from build123d import *

# Parameters (mm, degrees)
SKETCH1_W           = 50
SKETCH1_H           = 49.309999932
BOSS_EXTRUDE1_DEPTH = 22.098
SKETCH3_R           = 2.667
BOSS_EXTRUDE2_DEPTH = 14.098
SKETCH11_R          = 1.5875
CUT_EXTRUDE7_DEPTH  = 33.02
BOSS_EXTRUDE4_DEPTH = 2.54
SKETCH16_R          = 1.5875
CUT_EXTRUDE11_DEPTH = 2.54
BOSS_EXTRUDE5_DEPTH = 7
SKETCH21_R          = 3
CUT_EXTRUDE14_DEPTH = 7
BOSS_EXTRUDE6_DEPTH = 5


with BuildPart() as part:
    # Sketch1 → Boss-Extrude1 (new body)
    with BuildSketch(Plane.XY):
        with Locations((0, 0.745000034)):
            Rectangle(SKETCH1_W, SKETCH1_H)
        Polygon((12.5, 47.050635095), (-12.5, 47.050635095), (-25, 25.4), (25, 25.4), align=None)
    extrude(amount=BOSS_EXTRUDE1_DEPTH)

    # Sketch3 → Boss-Extrude2 (add)
    with BuildSketch(Plane(origin=(0, 0, 0), x_dir=(-1, 0, 0), z_dir=(0, 0, -1))):
        with BuildLine():
            ThreePointArc((-26.155685571, 27.78125), (-33.743775214, 30.924339642), (-30.600685571, 23.33625))
            Line((-30.600685571, 23.33625), (-25, 23.33625))
            Line((-25, 23.33625), (-25, 25.4))
            Line((-25, 25.4), (-23.625184671, 27.78125))
            Line((-23.625184671, 27.78125), (-26.155685571, 27.78125))
        make_face()
        with Locations((-30.600685571, 27.78125)):
            Circle(SKETCH3_R, mode=Mode.SUBTRACT)
    extrude(amount=-BOSS_EXTRUDE2_DEPTH)

    # Sketch11 → Cut-Extrude7 (cut)
    with BuildSketch(Plane.XY.offset(22.098)):
        with BuildLine():
            Line((-17.892329478, 22.025071278), (-19.92, 22.179409051))
            Line((-19.92, 22.179409051), (-19.92, -11.209999932))
            Line((-19.92, -11.209999932), (-18.65, -11.209999932))
            ThreePointArc((-18.65, -11.209999932), (-14.159871939, -13.069871871), (-12.3, -17.559999932))
            Line((-12.3, -17.559999932), (-12.3, -18.829999932))
            Line((-12.3, -18.829999932), (12.3, -18.829999932))
            Line((12.3, -18.829999932), (12.3, -17.559999932))
            ThreePointArc((12.3, -17.559999932), (14.159871939, -13.069871871), (18.65, -11.209999932))
            Line((18.65, -11.209999932), (19.92, -11.209999932))
            Line((19.92, -11.209999932), (19.92, 24.038818102))
            Line((19.92, 24.038818102), (18.060590949, 27.259409051))
            Line((18.060590949, 27.259409051), (9.567060633, 41.970635095))
            Line((9.567060633, 41.970635095), (-9.567060633, 41.970635095))
            Line((-9.567060633, 41.970635095), (-18.024928281, 27.321178603))
            ThreePointArc((-18.024928281, 27.321178603), (-12.880508254, 24.800266004), (-17.892329478, 22.025071278))
        make_face()
        with Locations((-16.11, 24.719409119)):
            Circle(SKETCH11_R)
        with Locations((16.11, -15.02)):
            Circle(SKETCH11_R)
        with Locations((-16.11, -15.019999932)):
            Circle(SKETCH11_R)
    extrude(amount=-CUT_EXTRUDE7_DEPTH, mode=Mode.SUBTRACT)

    # Sketch12 → Boss-Extrude4 (add)
    with BuildSketch(Plane(origin=(0, 0, 0), x_dir=(-1, 0, 0), z_dir=(0, 0, -1))):
        Polygon((-25, -23.909999932), (25, -23.909999932), (25, 25.4), (12.5, 47.050635095), (-12.5, 47.050635095), (-25, 25.4), align=None)
    extrude(amount=-BOSS_EXTRUDE4_DEPTH)

    # Sketch16 → Cut-Extrude11 (cut)
    with BuildSketch(Plane.XY.offset(2.54)):
        with Locations((-10.16, 6.35)):
            Circle(SKETCH16_R)
        with Locations((-10.16, -6.35)):
            Circle(SKETCH16_R)
        with Locations((10.16, 6.35)):
            Circle(SKETCH16_R)
        with Locations((10.16, -6.35)):
            Circle(SKETCH16_R)
    extrude(amount=-CUT_EXTRUDE11_DEPTH, mode=Mode.SUBTRACT)

    # Sketch20 → Boss-Extrude5 (add)
    with BuildSketch(Plane.XY.offset(2.54)):
        Polygon((-9.198279291, 25.191225954), (-6.198279291, 25.191225954), (-6.198279291, 26.191225954), (-8.198279291, 26.191225954), (-8.198279291, 27.391225954), (-6.198279291, 27.391225954), (-6.198279291, 28.391225954), (-9.198279291, 28.391225954), align=None)
        Polygon((8.198279291, 26.191225954), (8.198279291, 27.391225954), (6.198279291, 27.391225954), (6.198279291, 28.391225954), (9.198279291, 28.391225954), (9.198279291, 25.191225954), (6.198279291, 25.191225954), (6.198279291, 26.191225954), align=None)
    extrude(amount=BOSS_EXTRUDE5_DEPTH)

    # Sketch21 → Cut-Extrude14 (cut)
    with BuildSketch(Plane.XY.offset(2.54)):
        with Locations((0.698279291, 30.391225954)):
            Circle(SKETCH21_R)
    extrude(amount=-CUT_EXTRUDE14_DEPTH, mode=Mode.SUBTRACT)

    # Sketch22 → Boss-Extrude6 (add)
    with BuildSketch(Plane.XY.offset(2.54)):
        Polygon((4, 1.5), (-4, 1.5), (-4, 0.5), (-3, 0.5), (3, 0.5), (4, 0.5), align=None)
        Polygon((3, -0.5), (-3, -0.5), (-4, -0.5), (-4, -1.5), (4, -1.5), (4, -0.5), align=None)
    extrude(amount=BOSS_EXTRUDE6_DEPTH)


solid = part.part
Here's how the part is built. I have some questions about the finished solid (model axes, mm). A direction names the side the tool comes from. Round coordinates to 2 decimals unless told otherwise and drop trailing zeros. Order: outer loops, then holes, each group sorted by start corner. A loop starts at its lowest first (then second) coordinate and runs counter-clockwise, first axis right, second up. Notation, with made-up numbers: (-17.5, -4.75) -> (0.5, -4.75) arc R27 ccw to (0.5, 31.25) -> close; hole circle Ø3 at (60.25, 1.25). An arc over 180 degrees is marked (long way). Return JSON: item names as keys, results as strings.
Q1. If we section it at B-B on z = 1.75: Give the number of separate pieces and of enclosed holes in the cut face, plus the area to 3 significant figures.
Filled sheet:
{"separate pieces": "1", "enclosed holes": "6", "area": "3,270 mm^2"}
Q2. If we mould it in two halves opening along Y, with no side actions, what happens to faces 3 (the cylindrical face through (-12.884, 24.899, 12.456)), 4 (the flat face through (0, 47.051, 11))? For each: released by +Y, released by -Y, zero draft, split by the parting line, or undercut.
Filled sheet:
{"face 3": "undercut", "face 4": "released by +Y"}
Q3. If we section it at C-C on y = 10.5: List the corners of the cut face in (x, z) for me, plus the area to 3 significant figures.
Filled sheet:
{"outline": "(-25, 0) -> (25, 0) -> (25, 22.1) -> (19.92, 22.1) -> (19.92, 2.54) -> (-19.92, 2.54) -> (-19.92, 22.1) -> (-25, 22.1) -> close", "area": "326 mm^2"}
Q4. For pin 1 Ø0.8 at (y, z) = (-1, 6) entering from +X; pin 2 Ø3.5 at (x, y) = (-16.11, -15.02) entering from +Z; pin 3 Ø4.5 at (x, y) = (30.6, 27.78) entering from +Z; pin 4 Ø1.6 at (y, z) = (26.5, 4.5) entering from -X, each with a flat end and sliding along its axis, tell me the tip position at first contact or that it passes through.
Filled sheet:
{"pin 1": "stops at x = 25", "pin 2": "stops at z = 22.1", "pin 3": "passes through", "pin 4": "stops at x = -24.83"}
Q5. If we section it at A-A on y = -6.35: List the corners of the cut face in (x, z) for me.
Filled sheet:
{"outline": "(-25, 0) -> (-11.75, 0) -> (-11.75, 2.54) -> (-19.92, 2.54) -> (-19.92, 22.1) -> (-25, 22.1) -> close; (-8.57, 0) -> (8.57, 0) -> (8.57, 2.54) -> (-8.57, 2.54) -> close; (11.75, 0) -> (25, 0) -> (25, 22.1) -> (19.92, 22.1) -> (19.92, 2.54) -> (11.75, 2.54) -> close"}
Q6. Which directions (+Z, -Z, +X, -X, +Y, -Y) give clear straight access to the entire face, cutting with the end or side of a thin tool? Please do faces 1 (the cylindrical face through (-8.694, -6.958, 1.288)), 2 (the cylindrical face through (-14.644, -15.628, 12.456)).
Filled sheet:
{"face 1": "+Z, -Z", "face 2": "+Z"}
Q7. I need wall thicknesses on line 1 along Y through (x, z) = (-10.16, 0.9); line 2 along Y through (x, z) = (-8, 13.5); line 3 along X through (y, z) = (-8, 17). Which ranges of each line are inside material? Lowest first, please. Write a range as from..to.
Filled sheet:
{"line 1": "y = -23.91..-7.94, -4.76..4.76, 7.94..47.05", "line 2": "y = -23.91..-18.83, 41.97..47.05", "line 3": "x = -25..-19.92, 19.92..25"}
